from build123d import *

# Parameters (mm, degrees)
STOCK_SPINE_MASTER_1_START     = 21.5
STOCK_SPINE_MASTER_1_OUTLINE_R = 2.25
STOCK_SPINE_MASTER_1_DEPTH     = 3.2
FILLET1_R                      = 5
FILLET2_R                      = 2
FILLET3_R                      = 20
CUT_EXTRUDE4_DEPTH             = 199.32814828
FILLET4_R                      = 2
CUT_EXTRUDE6_DEPTH             = 199.328148417
LPATTERN2_COUNT                = 2
LPATTERN2_PITCH                = 18
LPATTERN2_COL_COUNT            = 2
LPATTERN2_COL_PITCH            = 18


# Read off the part's stored shape, not the designer's step: Stock-spine_master-1
with BuildPart() as part:
    # Stock-spine_master-1 outline → Stock-spine_master-1 (new body)
    with BuildSketch(Plane.YZ.offset(STOCK_SPINE_MASTER_1_START)):
        with BuildLine():
            Line((-174, -50.2), (-158, -50.2))
            Line((-158, -50.2), (-142, -13))
            Line((-142, -13), (-72.784271247, -13))
            ThreePointArc((-72.784271247, -13), (-64.365235735, -14.674650285), (-57.227922061, -19.443650814))
            Line((-57.227922061, -19.443650814), (-52.943650814, -23.727922061))
            ThreePointArc((-52.943650814, -23.727922061), (-47.104030535, -27.629831585), (-40.215728753, -29))
            Line((-40.215728753, -29), (-2, -29))
            Line((-2, -29), (-2, 13))
            Line((-2, 13), (-142, 13))
            Line((-142, 13), (-158, 95.12))
            Line((-158, 95.12), (-174, 95.12))
            Line((-174, 95.12), (-174, -50.2))
        make_face()
        with Locations((-166, -42.2)):
            Circle(STOCK_SPINE_MASTER_1_OUTLINE_R, mode=Mode.SUBTRACT)
        with Locations((-166, -26.2)):
            Circle(STOCK_SPINE_MASTER_1_OUTLINE_R, mode=Mode.SUBTRACT)
        with Locations((-166, 0)):
            Circle(STOCK_SPINE_MASTER_1_OUTLINE_R, mode=Mode.SUBTRACT)
        with Locations((-134, 0)):
            Circle(STOCK_SPINE_MASTER_1_OUTLINE_R, mode=Mode.SUBTRACT)
        with Locations((-65, 0)):
            Circle(STOCK_SPINE_MASTER_1_OUTLINE_R, mode=Mode.SUBTRACT)
        with Locations((-33, 0)):
            Circle(STOCK_SPINE_MASTER_1_OUTLINE_R, mode=Mode.SUBTRACT)
        with Locations((-166, 47.12)):
            Circle(STOCK_SPINE_MASTER_1_OUTLINE_R, mode=Mode.SUBTRACT)
        with Locations((-166, 71.12)):
            Circle(STOCK_SPINE_MASTER_1_OUTLINE_R, mode=Mode.SUBTRACT)
        with Locations((-166, 87.12)):
            Circle(STOCK_SPINE_MASTER_1_OUTLINE_R, mode=Mode.SUBTRACT)
    extrude(amount=STOCK_SPINE_MASTER_1_DEPTH)

    # Fillet1
    fillet1_edges = [part.edges().sort_by_distance(p)[0] for p in [
        (23.1, -158, 95.12),
        (23.1, -2, 13),
        (23.1, -2, -29),
        (23.1, -158, -50.2),
    ]]
    fillet(fillet1_edges, radius=FILLET1_R)

    # Fillet2
    fillet2_edges = [part.edges().sort_by_distance(p)[0] for p in [
        (23.1, -174, -50.2),
        (23.1, -174, 95.12),
    ]]
    fillet(fillet2_edges, radius=FILLET2_R)

    # Fillet3
    fillet3_edges = [part.edges().sort_by_distance(p)[0] for p in [
        (23.1, -142, 13),
        (23.1, -142, -13),
    ]]
    fillet(fillet3_edges, radius=FILLET3_R)

    # Sketch7 → Cut-Extrude4 (cut, through all)
    with BuildSketch(Plane(origin=(24.7, 0, 0), x_dir=(0, 0, -1), z_dir=(1, 0, 0))):
        with BuildLine():
            Line((-28.027740447, -151.040780627), (-40.87, -153.542925693))
            Line((-40.87, -153.542925693), (-40.87, -168))
            Line((-40.87, -168), (-13, -168))
            Line((-13, -168), (-13, -142.133906195))
            ThreePointArc((-13, -142.133906195), (-19.743434086, -147.887228617), (-28.027740447, -151.040780627))
        make_face()
        with BuildLine():
            Line((23, -8), (13, -8))
            Line((13, -8), (13, -55.463763172))
            ThreePointArc((13, -55.463763172), (14.063796748, -54.191923537), (15.201010127, -52.985281374))
            Line((15.201010127, -52.985281374), (19.485281374, -48.701010127))
            ThreePointArc((19.485281374, -48.701010127), (22.08655439, -44.807929941), (23, -40.215728753))
            Line((23, -40.215728753), (23, -8))
        make_face()
        with BuildLine():
            Line((13, -145.443926245), (13, -159.75))
            Line((13, -159.75), (39.083148267, -159.75))
            Line((39.083148267, -159.75), (22.727111066, -152.71514529))
            ThreePointArc((22.727111066, -152.71514529), (17.433060426, -149.655432834), (13, -145.443926245))
        make_face()
    extrude(amount=-CUT_EXTRUDE4_DEPTH, mode=Mode.SUBTRACT)

    # Fillet4
    fillet4_edges = [part.edges().sort_by_distance(p)[0] for p in [
        (23.1, -168, 13),
        (23.1, -168, 40.87),
        (23.1, -153.542925693, 40.87),
        (23.1, -142.133906195, 13),
        (23.1, -55.463763172, -13),
        (23.1, -145.443926245, -13),
        (23.1, -8, -13),
        (23.1, -159.75, -13),
        (23.1, -159.75, -39.083148267),
        (23.1, -8, -23),
    ]]
    fillet(fillet4_edges, radius=FILLET4_R)

    # Sketch10 → Cut-Extrude6 (cut, through all)
    with BuildSketch(Plane(origin=(24.7, 0, 0), x_dir=(0, 0, -1), z_dir=(1, 0, 0))):
        with BuildLine():
            Line((-7, -98.922649731), (3, -93.149147039))
            ThreePointArc((3, -93.149147039), (8.464101615, -94.613248654), (7, -100.077350269))
            Line((7, -100.077350269), (-3, -105.850852961))
            ThreePointArc((-3, -105.850852961), (-8.464101615, -104.386751346), (-7, -98.922649731))
        make_face()
    cut_extrude6 = extrude(amount=-CUT_EXTRUDE6_DEPTH, mode=Mode.SUBTRACT)

    # LPattern2: Cut-Extrude6 ×2
    with Locations(*[(0, i * LPATTERN2_PITCH, 0) for i in range(1, LPATTERN2_COUNT)]):
        add(cut_extrude6, mode=Mode.SUBTRACT)

    # LPattern2 col: Cut-Extrude6 ×2
    with Locations(*[(0, -i * LPATTERN2_COL_PITCH, 0) for i in range(1, LPATTERN2_COL_COUNT)]):
        add(cut_extrude6, mode=Mode.SUBTRACT)


solid = part.part
Work out the finished part from the listing and answer in its coordinate system (mm). A direction names the side the tool comes from. Give positions to 0.01 mm unless a question says otherwise; leave off trailing zeros. Write each loop counter-clockwise with the first axis right and the second up, starting at its lowest first coordinate (ties: lowest second). Pieces come first, ordered by that corner, then holes. Notation, with made-up numbers: (-8.75, -19) - (26.25, -19) arc R17 ccw to (26.25, 2) - close; hole circle Ø3 at (19, -14). An arc over 180 degrees is marked (long way). One line per item, written item: value. Start each with the question number.
1. Find section A-A (y = -33). Write down the section's boundary in (x, z), then the cut area to 3 significant figures.
2. Given pin 1 (1.5 mm diameter, centred on x = 24, y = -115.5, fed in from +Z); pin 2 (1.6 mm diameter, centred on x = 23, y = -153, fed in from -Z) (3 decimals), each flat-ended and moving along its own axis, determine where each tip first touches the part or whether it passes through.
3. For a pull along Z with two mould halves and no side action, classify faces 1 (the cylindrical face through (23.12, -122.46, 8.42)), 2 (the cylindrical face through (23.078, -64.477, -14.629)), 3 (the flat face through (23.1, -151.1, 59.7)) as +Z half, -Z half, draft (parallel to the pull), parting line (faces both ways), or undercut.
4. Find section D-D (y = -96). Write down the section's boundary in (x, z).
5. Find section B-B (z = 87.12). Write down the section's boundary in (x, y).
6. For faces 4 (the flat face through (24.7, -108, 12)), 5 (the flat face through (23.078, -55.116, -21.556)), 6 (the flat face through (23.122, -84.924, -2.07)), determine the directions among +Z, -Z, +X, -X, +Y, -Y from which every point of the face is accessible in a straight line to the end or side of a thin tool.
7. Consider probe 1 along Z at (x, y) = (22.8, -21.5); probe 2 along Z at (x, y) = (21.7, -159.5); probe 3 along Z at (x, y) = (22.45, -161). Determine where each line is inside the solid, lowest interval first.
8. Find section C-C (x = 22.7). State how many separate pieces and enclosed holes the cut face has, then the cut area to 3 significant figures.
Geometry results:
1. outline: (21.5, -29) - (24.7, -29) - (24.7, -23) - (21.5, -23) - close; (21.5, -13) - (24.7, -13) - (24.7, -2.25) - (21.5, -2.25) - close; (21.5, 2.25) - (24.7, 2.25) - (24.7, 13) - (21.5, 13) - close
1. area: 88.0 mm2
2. pin 1: z = 13
2. pin 2: z = -40.435
3. face 1: undercut
3. face 2: -Z half
3. face 3: +Z half
4. outline: (21.5, -13) - (24.7, -13) - (24.7, -8.95) - (21.5, -8.95) - close; (21.5, 1.94) - (24.7, 1.94) - (24.7, 13) - (21.5, 13) - close
5. outline: (21.5, -174) - (24.7, -174) - (24.7, -168.25) - (21.5, -168.25) - close; (21.5, -163.75) - (24.7, -163.75) - (24.7, -156.44) - (21.5, -156.44) - close
6. face 4: +Z, -Z, +X, +Y, -Y
6. face 5: -Z, +X, -X
6. face 6: +X, -X
7. probe 1: -29 to -23, -13 to 13
7. probe 2: -49.87 to -30.34, -14.03 to 13, 40.87 to 94.38
7. probe 3: -50.19 to 13, 40.87 to 94.99
8. separate pieces: 1
8. enclosed holes: 15
8. area: 6,650 mm2
